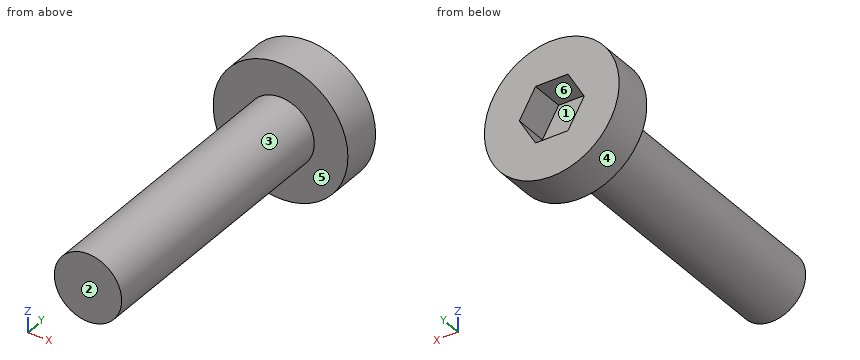
Solid Edge part; units mm, degrees
sketch "Sketch1" plane through (0, 0, 0) normal (0, -1, 0) x (1, 0, 0)
  circle A0 centre (0, 0) radius 6
extrude "Protrusion1" add sketch "Sketch1" along normal blind 3.6
sketch "Sketch2" plane through (0, -3.6, 0) normal (0, -1, 0) x (1, 0, 0)
  circle A0 centre (0, 0) radius 3
extrude "Protrusion2" add sketch "Sketch2" along normal blind 25
cosmetic_thread "Thread1"
sketch "Sketch3" plane through (0, 0, 0) normal (0, 1, 0) x (0, 0, -1)
  line L0 (2.5, -1.4434) -> (2.5, 1.4434)
  line L1 (2.5, 1.4434) -> (0, 2.8868)
  line L2 (0, 2.8868) -> (-2.5, 1.4434)
  line L3 (-2.5, 1.4434) -> (-2.5, -1.4434)
  line L4 (-2.5, -1.4434) -> (0, -2.8868)
  line L5 (0, -2.8868) -> (2.5, -1.4434)
extrude "ExtrudedCutout_4" cut sketch "Sketch3" against normal blind 3
properties material "Nylon, general purpose"
Geometry check sheet. Reference: the model listing, model coordinates, mm. Face numbers are marked on the shaded views. A direction names the side the tool comes from. Coordinates: 2 decimals unless noted, no trailing zeros. Write each loop counter-clockwise with the first axis right and the second up, starting at its lowest first coordinate (ties: lowest second). Pieces come first, ordered by that corner, then holes. Notation, with made-up numbers: M 34,-40 L 50,-40 A19 ccw 50,-6 Z; hole C -31.5,53 d8. An arc over 180 degrees is marked long. One line per item, written item: value. Start each with the question number.
(1) Tool access check on the marked faces 1, 2 and 3. Record the directions out of +Z, -Z, +X, -X, +Y, -Y that give a thin tool (end or side, any length) a straight path to the whole face; none if there is none.
(2) Depth check by flat-ended pin: pin 1 (1 mm diameter, centred on x = 3, y = -25, fed in from +Z); pin 2 (5.5 mm diameter, centred on x = 1.5, z = 1, fed in from +Y); pin 3 (1 mm diameter, centred on y = -14.5, z = 1, fed in from -X); pin 4 (4 mm diameter, centred on y = -7, z = -2.5, fed in from +X). Enter the tip coordinate at first touch or a pass-through.
(3) Sectioned sample at B-B, the plane y = -17.5. Enter the section's corners in (x, z), and give its area (3 significant figures).
(4) Sectioned sample at A-A, the plane x = 0. Enter the section's corners in (y, z), and give its area (3 significant figures).
(5) Sectioned sample at D-D, the plane z = 4.25. Enter the section's corners in (x, y).
(6) Sectioned sample at C-C, the plane z = 0.75. Enter the section's corners in (x, y).
(7) Scan lines: line 1 along Y through (x, z) = (-4.75, 2.75); line 2 along X through (y, z) = (-1.75, 0.5); line 3 along Y through (x, z) = (-1.25, 2.25). Record each from-to range of solid material in increasing order. Write a range as [from, to].
(8) Release check for a two-part mould opening along Z. For the marked faces 4, 5 and 6 record: released by +Z, released by -Z, zero draft, split by the parting line, or undercut.
Filled sheet:
1. face 1: +Y
1. face 2: +Z, -Z, +X, -X, -Y
1. face 3: -Y
2. pin 1: z = 1.66
2. pin 2: y = 0
2. pin 3: x = -2.96
2. pin 4: x = 2.96
3. outline: C 0,0 d6
3. area: 28.3 mm²
4. outline: M -28.6,-3 L -3.6,-3 L -3.6,-6 L 0,-6 L 0,-2.5 L -3,-2.5 L -3,2.5 L 0,2.5 L 0,6 L -3.6,6 L -3.6,3 L -28.6,3 Z
4. area: 178 mm²
5. outline: M -4.24,-3.6 L 4.24,-3.6 L 4.24,0 L -4.24,0 Z
6. outline: M -5.95,-3.6 L -2.9,-3.6 L -2.9,-28.6 L 2.9,-28.6 L 2.9,-3.6 L 5.95,-3.6 L 5.95,0 L 2.45,0 L 2.45,-3 L -2.45,-3 L -2.45,0 L -5.95,0 Z
7. line 1: [-3.6, 0]
7. line 2: [-5.98, -2.6], [2.6, 5.98]
7. line 3: [-28.6, -3]
8. face 4: split by the parting line
8. face 5: zero draft
8. face 6: undercut
